Model file for the job. Use its own axes, mm. Coordinates: 2 decimals unless noted, no trailing zeros. Order: outer loops, then holes, each group sorted by start corner. A loop starts at its lowest first (then second) coordinate and runs counter-clockwise, first axis right, second up. Notation, with made-up numbers: (-7.75, 64.25) - (32.25, 64.25) arc R16 ccw to (32.25, 77.25) - close; hole circle Ø6 at (35, -32). An arc over 180 degrees is marked (long way). Put each result on its own line as item: value. Start each with the question number.
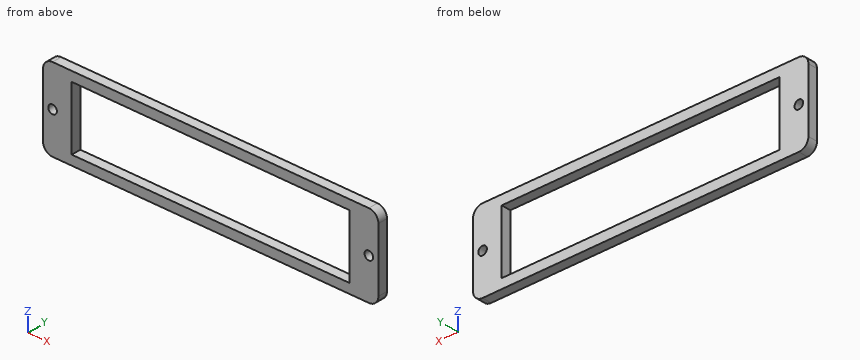
Autodesk Inventor part; units mm, degrees
ref_plane "YZ Plane" through (0, 0, 0) normal (1, 0, 0) x (0, 1, 0)
ref_plane "XZ Plane" through (0, 0, 0) normal (0, 1, 0) x (-1, 0, 0)
ref_plane "XY Plane" through (0, 0, 0) normal (0, 0, 1) x (1, 0, 0)
sketch "Sketch2" plane through (0, 0, 0) normal (0, 1, 0) x (-1, 0, 0)
  line L0 (72.5, 16.5) -> (-72.5, 16.5)
  line L1 (-72.5, 16.5) -> (-72.5, -16.5)
  line L2 (-72.5, -16.5) -> (72.5, -16.5)
  line L3 (72.5, -16.5) -> (72.5, 16.5)
  line L4 (72.5, 16.5) -> (-72.5, -16.5) construction
  line L5 (-72.5, 16.5) -> (72.5, -16.5) construction
  line L6 (87.5, -21.5) -> (-87.5, -21.5)
  line L7 (-87.5, -21.5) -> (-87.5, 21.5)
  line L8 (-87.5, 21.5) -> (87.5, 21.5)
  line L9 (87.5, 21.5) -> (87.5, -21.5)
  line L10 (87.5, -21.5) -> (-87.5, 21.5) construction
  line L11 (-87.5, -21.5) -> (87.5, 21.5) construction
  line L12 (72.5, 0) -> (82.5, 0) construction
  circle A0 centre (82.5, 0) radius 2.25
  line L13 (0, -16.5) -> (0, 16.5)
  circle A1 centre (-82.5, 0) radius 2.25
  point P0 (0, 0)
  dimension "d12" = 145
  dimension "d13" = 33
  dimension "d14" = 175
  dimension "d15" = 43
  dimension "d16" = 10
  dimension "d17" = 4.5
extrude "Extrusion2" add sketch "Sketch2" along normal blind 5
fillet "Fillet1" radius 5 1 edges at (87.5, 2.5, -21.5)
fillet "Fillet2" radius 5 3 edges at (87.5, 2.5, 21.5) (-87.5, 2.5, -21.5) (-87.5, 2.5, 21.5)
properties part number "Frame"
Item 1: Wall check: line 1 along Z through (x, y) = (32.5, 3.5); line 2 along Z through (x, y) = (82.5, 2.45); line 3 along X through (y, z) = (2.7, -1). Give the ranges that are in metal, low to high.
Item 2: Slice it at A-A, the plane z = 0. Give the cut face in (x, y).
Item 3: Slice it at B-B, the plane x = -66.5. Give the cut face in (y, z).
Item 4: Slice it at C-C, the plane y = 3.35. Give the cut face in (x, z), plus the area to 3 significant figures.
Here are the results:
1. line 1: z = -21.5 to -16.5, 16.5 to 21.5
1. line 2: z = -21.5 to -2.25, 2.25 to 21.5
1. line 3: x = -87.5 to -84.52, -80.48 to -72.5, 72.5 to 80.48, 84.52 to 87.5
2. outline: (-87.5, 0) - (-84.75, 0) - (-84.75, 5) - (-87.5, 5) - close; (-80.25, 0) - (-72.5, 0) - (-72.5, 5) - (-80.25, 5) - close; (72.5, 0) - (80.25, 0) - (80.25, 5) - (72.5, 5) - close; (84.75, 0) - (87.5, 0) - (87.5, 5) - (84.75, 5) - close
3. outline: (0, -21.5) - (5, -21.5) - (5, -16.5) - (0, -16.5) - close; (0, 16.5) - (5, 16.5) - (5, 21.5) - (0, 21.5) - close
4. outline: (-87.5, -16.5) arc R5 ccw to (-82.5, -21.5) - (82.5, -21.5) arc R5 ccw to (87.5, -16.5) - (87.5, 16.5) arc R5 ccw to (82.5, 21.5) - (-82.5, 21.5) arc R5 ccw to (-87.5, 16.5) - close; hole circle Ø4.5 at (-82.5, 0); hole (-72.5, -16.5) - (72.5, -16.5) - (72.5, 16.5) - (-72.5, 16.5) - close; hole circle Ø4.5 at (82.5, 0)
4. area: 2,690 mm^2
